```python
from build123d import *

# Parameters (mm, degrees)
F0_R     = 63.5
F0_R_2   = 3
F1_DEPTH = 19.05
F2_R     = 6.35


with BuildPart() as f1:
    # F0 (on Top) → F1 (new body)
    with BuildSketch(Plane.XY):
        Circle(F0_R)
        with BuildLine():
            ThreePointArc((38.1, -33.601042), (0, -50.8), (-38.1, -33.601042))
            ThreePointArc((-38.1, -33.601042), (-18.204557, -36.079269), (0, -27.679008))
            ThreePointArc((0, -27.679008), (18.204557, -36.079269), (38.1, -33.601042))
        make_face(mode=Mode.SUBTRACT)
        with BuildLine():
            ThreePointArc((-50.8, 0), (-35.149518, 24.490757), (-6.35, 20.576352))
            ThreePointArc((-6.35, 20.576352), (-11.076402, 10.766949), (-12.7, 0))
            ThreePointArc((-12.7, 0), (-11.076402, -10.766949), (-6.35, -20.576352))
            ThreePointArc((-6.35, -20.576352), (-35.149518, -24.490757), (-50.8, 0))
        make_face(mode=Mode.SUBTRACT)
        Circle(F0_R_2, mode=Mode.SUBTRACT)
        with BuildLine():
            ThreePointArc((6.35, -20.576352), (11.076402, -10.766949), (12.7, 0))
            ThreePointArc((12.7, 0), (11.076402, 10.766949), (6.35, 20.576352))
            ThreePointArc((6.35, 20.576352), (35.149518, 24.490757), (50.8, 0))
            ThreePointArc((50.8, 0), (35.149518, -24.490757), (6.35, -20.576352))
        make_face(mode=Mode.SUBTRACT)
        with BuildLine():
            ThreePointArc((38.1, 33.601042), (18.204557, 36.079269), (0, 27.679008))
            ThreePointArc((0, 27.679008), (-18.204557, 36.079269), (-38.1, 33.601042))
            ThreePointArc((-38.1, 33.601042), (0, 50.8), (38.1, 33.601042))
        make_face(mode=Mode.SUBTRACT)
    extrude(amount=F1_DEPTH)

    # F2
    f2_edges = [f1.edges().sort_by_distance(p)[0] for p in [
        (63.5, 0, 9.525),
        (-63.5, 0, 0),
        (-63.5, 0, 19.05),
    ]]
    fillet(f2_edges, radius=F2_R)


solid = f1.part
```
Geometry check sheet. Reference: the model listing, model coordinates, mm. Coordinates: 2 decimals unless noted, no trailing zeros. Use one line per item in the form item = value. Start each with the question number.
1) Go/stop test with flat-tipped pins: pin 1 Ø8 at (x, z) = (33.5, 13) entering from +Y; pin 2 Ø1.5 at (x, z) = (-10.5, 11.5) entering from +Y; pin 3 Ø7 at (x, y) = (0, 0) entering from +Z; pin 4 Ø10 at (y, z) = (33.5, 11) entering from -X. Record where each tip stops, or that it passes through.
2) Release check for a two-part mould opening along X. For faces 1 (the cylindrical face through (17.924, -36.035, 9.392)), 2 (the flat face through (12, 1, 0)), 3 (the cylindrical face through (-13.77, -61.99, 9.48)), 4 (the cylindrical face through (-3, 0, 9)) record: pulls with the +X half, pulls with the -X half, needs draft (parallel to the pull), parting line crosses it, or undercut.
3) Section check A-A on z = 14.5. State how many separate pieces and enclosed holes the cut face has, and give its area (3 significant figures).
4) Thickness scan on probe 1 along Y at (x, z) = (1, 12); probe 2 along Y at (x, z) = (-33, 12.75); probe 3 along Y at (x, z) = (9.5, 1.25). Record the ranges inside material, lowest first. Write a range as from..to.
Responses:
q1.pin_1 = 56.23
q1.pin_2 = 62.75
q1.pin_3 = 19.05
q1.pin_4 = -56.75
q2.face_1 = undercut
q2.face_2 = needs draft
q2.face_3 = parting line crosses it
q2.face_4 = undercut
q3.separate_pieces = 1
q3.enclosed_holes = 5
q3.area = 7,170 mm2
q4.probe_1 = -63.49..-50.79, -28.51..-2.83, 2.83..28.51, 50.79..63.49
q4.probe_2 = -54.25..-38.62, -35.34..-25.38, 25.38..35.34, 38.62..54.25
q4.probe_3 = -60.19..-49.9, -33.59..-22.88, -14.95..14.95, 22.88..33.59, 49.9..60.19
